Can you work these out from the model? Positions are in its coordinate system, mm. A direction names the side the tool comes from. Give positions to 0.01 mm unless a question says otherwise; leave off trailing zeros. Write each loop counter-clockwise with the first axis right and the second up, starting at its lowest first coordinate (ties: lowest second). Pieces come first, ordered by that corner, then holes.
from build123d import *

# Parameters (mm, degrees)
EXTRUDE_1_DEPTH     = 50
CUT_EXTRUDE_1_DEPTH = 173.916164658
SKETCH_3_W          = 20
SKETCH_3_H          = 20
CUT_EXTRUDE_2_DEPTH = 20
SKETCH_5_W          = 10
SKETCH_5_H          = 5
CUT_EXTRUDE_3_DEPTH = 173.916164658


with BuildPart() as part:
    # Эскиз1 → Бобышка-Вытянуть1 (new body)
    with BuildSketch(Plane.XY):
        Polygon((-150, 0), (-30, 0), (-30, 70), (-15, 50), (0, 70), (0, 0), (-30, -30), (-150, -30), align=None)
    extrude(amount=EXTRUDE_1_DEPTH)

    # Эскиз2 → Вырез-Вытянуть1 (cut, through all)
    with BuildSketch(Plane.XY.offset(50)):
        Polygon((-105, -30), (-75, -15), (-45, -30), align=None)
    extrude(amount=-CUT_EXTRUDE_1_DEPTH, mode=Mode.SUBTRACT)

    # Эскиз3 → Вырез-Вытянуть2 (cut)
    with BuildSketch(Plane.XY.offset(50)):
        with Locations((-75, -10)):
            Rectangle(SKETCH_3_W, SKETCH_3_H)
    extrude(amount=-CUT_EXTRUDE_2_DEPTH, mode=Mode.SUBTRACT)

    # Эскиз5 → Вырез-Вытянуть3 (cut, through all)
    with BuildSketch(Plane(origin=(0, 0, 0), x_dir=(1, 0, 0), z_dir=(0, 1, 0))):
        with Locations((-145, -2.5)):
            Rectangle(SKETCH_5_W, SKETCH_5_H)
        with Locations((-145, -47.5)):
            Rectangle(SKETCH_5_W, SKETCH_5_H)
    extrude(amount=-CUT_EXTRUDE_3_DEPTH, mode=Mode.SUBTRACT)


solid = part.part
(1) Imagine slicing it at D-D, the plane y = -12. Write out the boundary of the cut face in (x, z).
Returned:
outline: (-150, 5) - (-140, 5) - (-140, 0) - (-12, 0) - (-12, 50) - (-65, 50) - (-65, 30) - (-85, 30) - (-85, 50) - (-140, 50) - (-140, 45) - (-150, 45) - close
(2) Imagine slicing it at A-A, the plane z = 36.5. Write out the boundary of the cut face in (x, y).
Returned:
outline: (-150, -30) - (-105, -30) - (-85, -20) - (-85, 0) - (-150, 0) - close; (-65, -20) - (-45, -30) - (-30, -30) - (0, 0) - (0, 70) - (-15, 50) - (-30, 70) - (-30, 0) - (-65, 0) - close
(3) Will these pins go through, and if not, where does the flat tip stop? P1, Ø12, axis at y = 23.5, z = 7, coming from the -X side; P2, Ø15, axis at x = -67.5, z = 15, coming from the +Y side; P3, Ø8, axis at x = -146, y = -15, coming from the +Z side.
Returned:
P1: stops at x = -30
P2: stops at y = 0
P3: stops at z = 45
(4) If we mould it in two halves opening along X, with no side actions, what happens to faces 1 (the face through (0, 35, 25)), 2 (the face through (-57, -24, 25)), 3 (the face through (-145, -15, 45))? For each: +X half, -X half, draft (parallel to the pull), parting line (faces both ways), or undercut.
Returned:
face 1: +X half
face 2: undercut
face 3: draft
(5) If I drill on L1, parallel to X at y = 61, z = 30; L2, parallel to X at y = 55.5, z = 8 (3 decimals); L3, parallel to X at y = 34.5, z = 37.5, over which ranges is the centre line in solid material (lowest first)?
Returned:
L1: x = -30 to -23.25, -6.75 to 0
L2: x = -30 to -19.125, -10.875 to 0
L3: x = -30 to 0
(6) For faces 4 (the face through (-140, -15, 3)), 5 (the face through (-30, 35, 25)), 6 (the face through (-22.605, 60.14, 24.65)), which set-ups out of +Z, -Z, +X, -X, +Y, -Y let a thin tool reach every point of the face, with its end or its side?
Returned:
face 4: -Z, -X, +Y, -Y
face 5: +Z, -Z, -X, +Y
face 6: +Z, -Z, +Y
(7) Imagine slicing it at B-B, the plane y = 54. Write out the boundary of the cut face in (x, z).
Returned:
outline: (-30, 0) - (-18, 0) - (-18, 50) - (-30, 50) - close; (-12, 0) - (0, 0) - (0, 50) - (-12, 50) - close
(8) Imagine slicing it at C-C, the plane x = -88. Write out the boundary of the cut face in (y, z).
Returned:
outline: (-21.5, 0) - (0, 0) - (0, 50) - (-21.5, 50) - close
